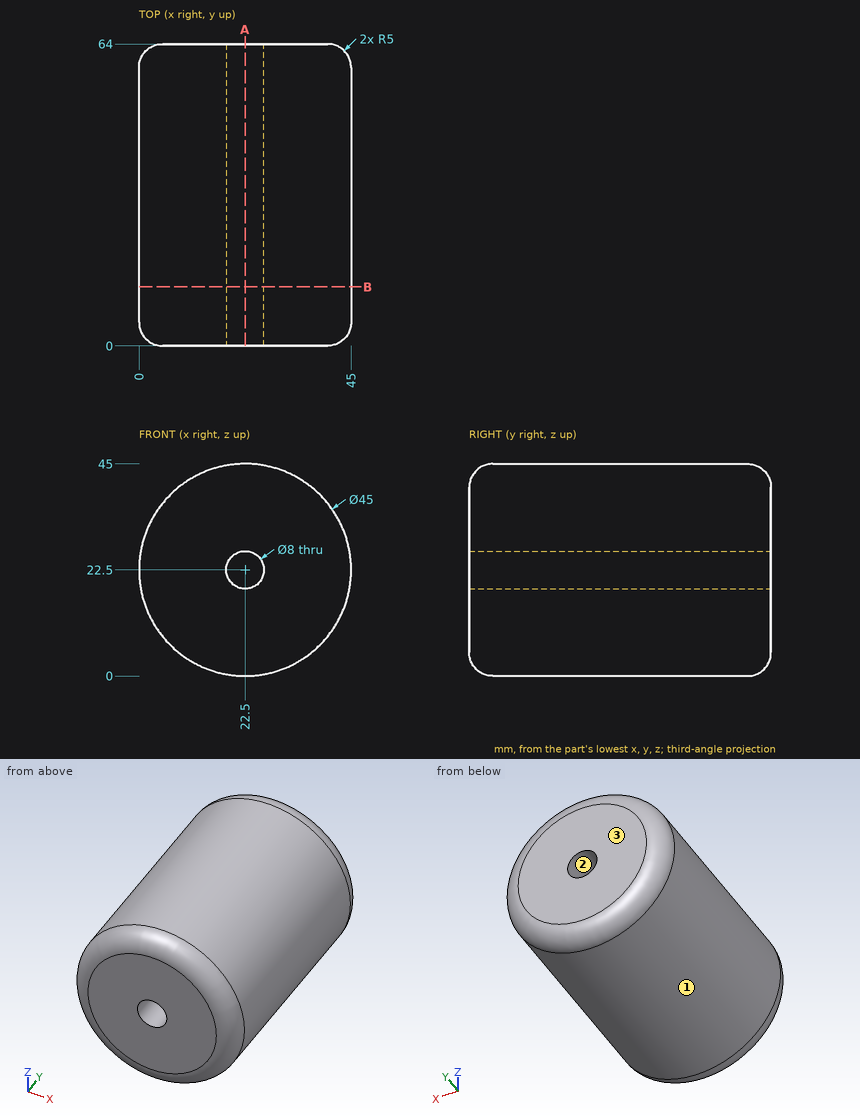
For this review, use the dimensioned drawing (mm, ordinates from the lowest corner) and the shaded views. Coordinates: 2 decimals unless noted, no trailing zeros. Order: outer loops, then holes, each group sorted by start corner. A loop starts at its lowest first (then second) coordinate and runs counter-clockwise, first axis right, second up. Notation, with made-up numbers: (32, 62.5) - (68, 62.5) arc R12 cw to (68, 80.5) - close; hole circle Ø2 at (-38.5, 44.25). An arc over 180 degrees is marked (long way). Answer as a JSON object with one key per item and string values. Group by question number.
1. Clearance check with flat-ended pins moving along their axes: P1, Ø1, axis at x = 29.5, y = 34, coming from the +Z side; P2, Ø2, axis at x = 27, y = 35.5, coming from the -Z side; P3, Ø2, axis at y = 33, z = 30.5, coming from the -X side. State where each tip first meets the part, or that it passes through.
2. The part is to be moulded in two halves that separate along Z. For the marked faces 1, 2 and 3, say which applies: pulls with the +Z half, pulls with the -Z half, needs draft (parallel to the pull), parting line crosses it, or undercut.
3. We need section A-A on x = 22.5. State the section outline as (y, z) points, then the cut area to 3 significant figures.
4. For probe 1 along Z at (x, y) = (22.5, 23); probe 2 along X at (y, z) = (28.5, 23); probe 3 along Z at (x, y) = (20, 7.5), list the stretches that pass through material, from the lowest coordinate up.
5. We need section B-B on y = 12.5. State the section outline as (x, z) points.
Final values:
{
 "1": {"P1": "z = 44.04", "P2": "z = 0.27", "P3": "x = 1.12"},
 "2": {"face 1": "parting line crosses it", "face 2": "undercut", "face 3": "needs draft"},
 "3": {"outline": "(0, 5) arc R5 ccw to (5, 0) - (59, 0) arc R5 ccw to (64, 5) - (64, 18.5) - (0, 18.5) - close; (0, 26.5) - (64, 26.5) - (64, 40) arc R5 ccw to (59, 45) - (5, 45) arc R5 ccw to (0, 40) - close", "area": "2,350 mm²"},
 "4": {"probe 1": "0 to 18.5, 26.5 to 45", "probe 2": "0.01 to 18.53, 26.47 to 44.99", "probe 3": "0.14 to 19.38, 25.62 to 44.86"},
 "5": {"outline": "circle Ø45 at (22.5, 22.5); hole circle Ø8 at (22.5, 22.5)"}
}
